```python
from build123d import *

# Parameters (mm, degrees)
PAD_DEPTH       = 24
POCKET_DEPTH    = 21
POCKET003_DEPTH = 1
POCKET004_DEPTH = 1
POCKET005_DEPTH = 5
SKETCH015_W     = 6
SKETCH015_H     = 11
SKETCH015_W_2   = 8
PAD006_DEPTH    = 12.5
SKETCH012_W     = 4
SKETCH012_H     = 4
SKETCH012_W_2   = 5
PAD007_DEPTH    = 21
POCKET006_DEPTH = 1
SKETCH016_R     = 1.7
HOLE_DEPTH      = 12.5
SKETCH017_R     = 1.7
HOLE001_DEPTH   = 21
CHAMFER_SIZE    = 1
SKETCH018_W     = 38
SKETCH018_H     = 39
PAD008_DEPTH    = 2.5


with BuildPart() as part:
    # Sketch → Pad (new body)
    with BuildSketch(Plane.XY):
        Polygon((-3, -6), (70, -6), (78, -16), (108, -16), (108, 70), (-3, 70), align=None)
    extrude(amount=PAD_DEPTH)

    # Sketch001 (on Face8 of Pad) → Pocket (cut)
    with BuildSketch(Plane.XY.offset(24)):
        Polygon((0, 67), (0, -3), (71, -3), (79, -13), (105, -13), (105, 67), align=None)
    extrude(amount=-POCKET_DEPTH, mode=Mode.SUBTRACT)

    # Sketch008 → Pocket003 (cut)
    with BuildSketch(Plane(origin=(0, 0, 0), x_dir=(1, 0, 0), z_dir=(0, 0, -1))):
        with BuildLine():
            ThreePointArc((91, 10), (88.5, 12.5), (86, 10))
            Line((86, 10), (86, -70))
            Line((86, -70), (91, -70))
            Line((91, 10), (91, -70))
        make_face()
        with BuildLine():
            ThreePointArc((101, 10), (98.5, 12.5), (96, 10))
            Line((96, 10), (96, -70))
            Line((96, -70), (101, -70))
            Line((101, 10), (101, -70))
        make_face()
        with BuildLine():
            ThreePointArc((71, 0), (68.5, 2.5), (66, 0))
            Line((66, 0), (66, -70))
            Line((66, -70), (71, -70))
            Line((71, 0), (71, -70))
        make_face()
        with BuildLine():
            ThreePointArc((81, 5), (78.5, 7.5), (76, 5))
            Line((76, 5), (76, -70))
            Line((76, -70), (81, -70))
            Line((81, 5), (81, -70))
        make_face()
        with BuildLine():
            ThreePointArc((41, 0), (38.5, 2.5), (36, 0))
            Line((36, 0), (36, -70))
            Line((36, -70), (41, -70))
            Line((41, 0), (41, -70))
        make_face()
        with BuildLine():
            ThreePointArc((61, 0), (58.5, 2.5), (56, 0))
            Line((56, 0), (56, -70))
            Line((56, -70), (61, -70))
            Line((61, 0), (61, -70))
        make_face()
        with BuildLine():
            ThreePointArc((31, 0), (28.5, 2.5), (26, 0))
            Line((26, 0), (26, -70))
            Line((26, -70), (31, -70))
            Line((31, 0), (31, -70))
        make_face()
        with BuildLine():
            ThreePointArc((21, 0), (18.5, 2.5), (16, 0))
            Line((16, 0), (16, -70))
            Line((16, -70), (21, -70))
            Line((21, 0), (21, -70))
        make_face()
        with BuildLine():
            ThreePointArc((51, 0), (48.5, 2.5), (46, 0))
            Line((46, 0), (46, -70))
            Line((46, -70), (51, -70))
            Line((51, 0), (51, -70))
        make_face()
        with BuildLine():
            ThreePointArc((11, 0), (8.5, 2.5), (6, 0))
            Line((6, 0), (6, -70))
            Line((6, -70), (11, -70))
            Line((11, 0), (11, -70))
        make_face()
    extrude(amount=-POCKET003_DEPTH, mode=Mode.SUBTRACT)

    # Sketch009 (on Face6 of Pocket003) → Pocket004 (cut)
    with BuildSketch(Plane(origin=(0, 70, 0), x_dir=(-1, 0, 0), z_dir=(0, 1, 0))):
        with BuildLine():
            ThreePointArc((-96, 18), (-98.5, 20.5), (-101, 18))
            Line((-101, 18), (-101, 0))
            Line((-101, 0), (-96, 0))
            Line((-96, 18), (-96, 0))
        make_face()
        with BuildLine():
            ThreePointArc((-86, 18), (-88.5, 20.5), (-91, 18))
            Line((-91, 18), (-91, 0))
            Line((-91, 0), (-86, 0))
            Line((-86, 18), (-86, 0))
        make_face()
        with BuildLine():
            ThreePointArc((-56, 18), (-58.5, 20.5), (-61, 18))
            Line((-61, 18), (-61, 0))
            Line((-61, 0), (-56, 0))
            Line((-56, 18), (-56, 0))
        make_face()
        with BuildLine():
            ThreePointArc((-76, 18), (-78.5, 20.5), (-81, 18))
            Line((-81, 18), (-81, 0))
            Line((-81, 0), (-76, 0))
            Line((-76, 18), (-76, 0))
        make_face()
        with BuildLine():
            ThreePointArc((-46, 18), (-48.5, 20.5), (-51, 18))
            Line((-51, 18), (-51, 0))
            Line((-51, 0), (-46, 0))
            Line((-46, 18), (-46, 0))
        make_face()
        with BuildLine():
            ThreePointArc((-36, 18), (-38.5, 20.5), (-41, 18))
            Line((-41, 18), (-41, 0))
            Line((-41, 0), (-36, 0))
            Line((-36, 18), (-36, 0))
        make_face()
        with BuildLine():
            ThreePointArc((-26, 18), (-28.5, 20.5), (-31, 18))
            Line((-31, 18), (-31, 0))
            Line((-31, 0), (-26, 0))
            Line((-26, 18), (-26, 0))
        make_face()
        with BuildLine():
            ThreePointArc((-16, 18), (-18.5, 20.5), (-21, 18))
            Line((-21, 18), (-21, 0))
            Line((-21, 0), (-16, 0))
            Line((-16, 18), (-16, 0))
        make_face()
        with BuildLine():
            ThreePointArc((-6, 18), (-8.5, 20.5), (-11, 18))
            Line((-11, 18), (-11, 0))
            Line((-11, 0), (-6, 0))
            Line((-6, 18), (-6, 0))
        make_face()
        with BuildLine():
            ThreePointArc((-66, 18), (-68.5, 20.5), (-71, 18))
            Line((-71, 18), (-71, 0))
            Line((-71, 0), (-66, 0))
            Line((-66, 18), (-66, 0))
        make_face()
    extrude(amount=-POCKET004_DEPTH, mode=Mode.SUBTRACT)

    # Sketch014 (on Face38 of Pocket003) → Pocket005 (cut)
    with BuildSketch(Plane.YZ.offset(108)):
        with BuildLine():
            ThreePointArc((0.25908, 9.405), (-3, 21.475), (-6.25908, 9.405))
            Line((-6.25908, 9.405), (0.25908, 9.405))
        make_face()
        with BuildLine():
            ThreePointArc((60.25908, 9.405), (57, 21.475), (53.74092, 9.405))
            Line((53.74092, 9.405), (60.25908, 9.405))
        make_face()
        with BuildLine():
            ThreePointArc((37.746425, 7.2), (36, 13.3), (34.253575, 7.2))
            Line((37.746425, 7.2), (34.253575, 7.2))
        make_face()
        with BuildLine():
            ThreePointArc((12.65, 12.069556), (18, 8.9), (23.35, 12.069556))
            Line((23.35, 17.930444), (23.35, 12.069556))
            ThreePointArc((23.35, 17.930444), (18, 21.1), (12.65, 17.930444))
            Line((12.65, 17.930444), (12.65, 12.069556))
        make_face()
    extrude(amount=-POCKET005_DEPTH, mode=Mode.SUBTRACT)

    # Sketch015 → Pad006 (join)
    with BuildSketch(Plane.XY.offset(3)):
        with Locations((3, 61.5)):
            Rectangle(SKETCH015_W, SKETCH015_H)
        with Locations((78, 61.5)):
            Rectangle(SKETCH015_W_2, SKETCH015_H)
    extrude(amount=PAD006_DEPTH)

    # Sketch012 → Pad007 (join)
    with BuildSketch(Plane.XY.offset(3)):
        with Locations((2, 65)):
            Rectangle(SKETCH012_W, SKETCH012_H)
        with Locations((87.5, 65)):
            Rectangle(SKETCH012_W_2, SKETCH012_H)
        with Locations((87.5, -11)):
            Rectangle(SKETCH012_W_2, SKETCH012_H)
        with Locations((2, -1)):
            Rectangle(SKETCH012_W, SKETCH012_H)
    extrude(amount=PAD007_DEPTH)

    # Sketch006 → Pocket006 (cut)
    with BuildSketch(Plane.XY.offset(24)):
        Polygon((-2, 69), (107, 69), (107, -15), (78.3, -15), (70.3, -5), (-2, -5), align=None)
        Polygon((-1, 68), (106, 68), (106, -14), (78.6, -14), (70.6, -4), (-1, -4), align=None, mode=Mode.SUBTRACT)
    extrude(amount=-POCKET006_DEPTH, mode=Mode.SUBTRACT)

    # Sketch016 (on Face8 of Pocket006) → Hole (cut)
    with BuildSketch(Plane.XY.offset(15.5)):
        with Locations((3.25, 59)):
            Circle(SKETCH016_R)
        with Locations((77, 59)):
            Circle(SKETCH016_R)
    extrude(amount=-HOLE_DEPTH, mode=Mode.SUBTRACT)

    # Sketch017 (on Face56 of Hole) → Hole001 (cut)
    with BuildSketch(Plane.XY.offset(24)):
        with Locations((1.5, 65.5)):
            Circle(SKETCH017_R)
        with Locations((87.5, 65.5)):
            Circle(SKETCH017_R)
        with Locations((87.5, -11.5)):
            Circle(SKETCH017_R)
        with Locations((1.5, -1.5)):
            Circle(SKETCH017_R)
    extrude(amount=-HOLE001_DEPTH, mode=Mode.SUBTRACT)

    # Chamfer
    chamfer_edges = [part.edges().sort_by_distance(p)[0] for p in [
        (-3, 70, 12),
        (-3, -6, 12),
        (-3, 32, 0),
        (33.5, -6, 0),
        (1.5, 70, 0),
        (8.5, 69, 1),
        (13.5, 70, 0),
        (18.5, 69, 1),
        (23.5, 70, 0),
        (33.5, 70, 0),
        (28.5, 69, 1),
        (104.5, 70, 0),
        (108, 70, 12),
        (98.5, 69, 1),
        (93.5, 70, 0),
        (88.5, 69, 1),
        (83.5, 70, 0),
        (78.5, 69, 1),
        (73.5, 70, 0),
        (68.5, 69, 1),
        (63.5, 70, 0),
        (58.5, 69, 1),
        (53.5, 70, 0),
        (48.5, 69, 1),
        (43.5, 70, 0),
        (38.5, 69, 1),
        (108, 27, 0),
        (108, -16, 12),
        (93, -16, 0),
        (74, -11, 0),
    ]]
    chamfer(chamfer_edges, length=CHAMFER_SIZE)

    # Sketch018 (on Face93 of Chamfer) → Pad008 (join)
    with BuildSketch(Plane.XY.offset(3)):
        with Locations((40, 23.5)):
            Rectangle(SKETCH018_W, SKETCH018_H)
    extrude(amount=PAD008_DEPTH)


with BuildPart() as part_1:
    # Body placement: moved
    add(part.part.moved(Location((0, 0, -2.5))))


solid = part_1.part
```
Geometry check sheet. Reference: the model listing, model coordinates, mm. A direction names the side the tool comes from. Coordinates: 2 decimals unless noted, no trailing zeros. Order: outer loops, then holes, each group sorted by start corner. A loop starts at its lowest first (then second) coordinate and runs counter-clockwise, first axis right, second up.
Item 1: Section check A-A (x = 8.5). Enter the section's corners in (y, z).
Item 2: Mould release check, pull along Y, two halves, no side actions. Record for faces 1 (the flat face through (66, 35, -2)), 2 (the flat face through (3, 62, 13)), 3 (the cylindrical face through (38.6, -2.5, -2)): released by +Y, released by -Y, zero draft, split by the parting line, or undercut.
Item 3: Depth check by flat-ended pin: pin 1 (6 mm diameter, centred on x = 83, y = -5.5, fed in from +Z); pin 2 (2.5 mm diameter, centred on x = 68.5, z = 9.5, fed in from +Y); pin 3 (0.5 mm diameter, centred on x = 50.5, z = 21, fed in from -Y). Enter the tip coordinate at first touch or a pass-through.
Item 4: Tool access check on faces 4 (the flat face through (48, 32, -1.5)), 5 (the flat face through (45, 67, 11)), 6 (the flat face through (107, 23.35, 13)). Record the directions out of +Z, -Z, +X, -X, +Y, -Y that give a thin tool (end or side, any length) a straight path to the whole face; none if there is none.
Item 5: Scan lines: line 1 along X through (y, z) = (63.5, 9.5); line 2 along X through (y, z) = (65.5, 11); line 3 along Y through (x, z) = (87.5, 5.5). Record each from-to range of solid material in increasing order.
Check sheet entries:
1. outline: (-6, -1.5) - (-5, -2.5) - (-2.5, -2.5) - (-2.5, -1.5) - (68, -1.5) - (69, -0.5) - (69, 18) - (70, 18) - (70, 21.5) - (69, 21.5) - (69, 20.5) - (68, 20.5) - (68, 21.5) - (67, 21.5) - (67, 0.5) - (-3, 0.5) - (-3, 21.5) - (-4, 21.5) - (-4, 20.5) - (-5, 20.5) - (-5, 21.5) - (-6, 21.5) - close
2. face 1: zero draft
2. face 2: undercut
2. face 3: released by +Y
3. pin 1: stops at z = 0.5
3. pin 2: stops at y = 69
3. pin 3: stops at y = -6
4. face 4: -Z, +Y
4. face 5: +Z
4. face 6: +X
5. line 1: x = -3 to 6, 74 to 82, 85 to 90, 105 to 108
5. line 2: x = -3 to -0.2, 3.2 to 6, 74 to 82, 85 to 85.8, 89.2 to 90, 105 to 108
5. line 3: y = -16 to -13.2, -9.8 to -9, 63 to 63.8, 67.2 to 69
